Input: part model. Units: mm. Frame: model coordinates. A direction names the side the tool comes from. Give positions to 0.01 mm unless a question says otherwise; leave off trailing zeros. Write each loop counter-clockwise with the first axis right and the second up, starting at its lowest first coordinate (ties: lowest second). Pieces come first, ordered by that corner, then holes. Notation, with made-up numbers: (-33.5, -13.75) - (21.5, -13.75) arc R28 ccw to (21.5, 18.25) - close; hole circle Ø3 at (51.5, 89). An arc over 180 degrees is marked (long way). Answer as CSV lines item,"result". Start each with the question number.
from build123d import *

# Parameters (mm, degrees)
PAD_DEPTH       = 3.95
PAD001_DEPTH    = 8
SKETCH003_W     = 50
SKETCH003_H     = 9.8
PAD002_DEPTH    = 1.5
CHAMFER_SIZE    = 2.5
CHAMFER001_SIZE = 5
FILLET_R        = 2.5
FILLET001_R     = 0.5


with BuildPart() as part:
    # Sketch → Pad (new body)
    with BuildSketch(Plane.XY):
        Polygon((-45, 19.75), (-45, -19.75), (-24.75, -19.75), (-24.75, -45), (-7.25, -45), (-7.25, 19.75), align=None)
    extrude(amount=PAD_DEPTH)

    # Sketch002 → Pad001 (join)
    with BuildSketch(Plane.XY):
        Polygon((-45, 20), (-55, 20), (-55, 0), (-149, 0), (-149, -70), (-7, -70), (-7, -45), (-45, -45), align=None)
    extrude(amount=PAD001_DEPTH)

    # Sketch003 (on Face7 of Pad001) → Pad002 (join)
    with BuildSketch(Plane.XY.offset(8)):
        with Locations((-114, -55)):
            Rectangle(SKETCH003_W, SKETCH003_H)
    extrude(amount=PAD002_DEPTH)

    # Chamfer
    chamfer_edges = [part.edges().sort_by_distance(p)[0] for p in [
        (-7.25, 19.75, 1.975),
    ]]
    chamfer(chamfer_edges, length=CHAMFER_SIZE)

    # Chamfer001
    chamfer001_edges = [part.edges().sort_by_distance(p)[0] for p in [
        (-55, 20, 4),
    ]]
    chamfer(chamfer001_edges, length=CHAMFER001_SIZE)

    # Fillet
    fillet_edges = [part.edges().sort_by_distance(p)[0] for p in [
        (-55, 0, 4),
        (-149, 0, 4),
        (-149, -70, 4),
        (-7, -70, 4),
    ]]
    fillet(fillet_edges, radius=FILLET_R)

    # Fillet001
    fillet001_edges = [part.edges().sort_by_distance(p)[0] for p in [
        (-114, -59.9, 9.5),
        (-89, -55, 9.5),
        (-114, -50.1, 9.5),
        (-139, -55, 9.5),
    ]]
    fillet(fillet001_edges, radius=FILLET001_R)


solid = part.part
1) Reachability of faces 5 (the flat face through (-101, 0, 4)), 6 (the flat face through (-24.75, -32, 2)), 7 (the flat face through (-27, 19.75, 2)), 8 (the flat face through (-45, -20, 5)), 9 (the flat face through (-26, -5, 3.95)) from +Z, -Z, +X, -X, +Y, -Y: full face, straight path, thin tool, end or side. Return the list, or none.
2) Material intervals for line 1 (X direction, y = -26, z = 2.25); line 2 (Y direction, x = -27.5, z = 0.5); line 3 (Y direction, x = -30.5, z = 4.5), sorted ascending. Write a range as from..to.
3) Contact query for flat-ended pins moving along their axis: P1, Ø3, axis at x = -96.5, z = 7, coming from the +Y side; P2, Ø1.2, axis at y = -15.5, z = 3, coming from the +X side; P3, Ø4.5, axis at x = -32.5, z = 2, coming from the +Y side. Output: stop coordinate, or through.
4) Cut plane D-D on x = -135. Output: boundary loops of the cut face in (y, z), and give its area (3 significant figures).
5) Cut plane B-B on y = -26. Output: boundary loops of the cut face in (x, z), and give its area (3 significant figures).
6) Cut plane C-C on z = 1.75. Output: boundary loops of the cut face in (x, y), and give its area (3 significant figures).
7) Cut plane A-A on x = -37.5. Output: boundary loops of the cut face in (y, z), and give its area (3 significant figures).
8) Pull-direction query (Y, two-part tool) for faces 1 (the flat face through (-79, -70, 4)), 2 (the flat face through (-7, -56, 4)), 3 (the flat face through (-53, 17, 4)), 4 (the flat face through (-35, -19.75, 2)); classes: +Y half, -Y half, draft (parallel to the pull), parting line (faces both ways), or undercut.
Numbers:
1,face 5,"+Z, -Z, -X, +Y"
1,face 6,"+Z, -Z"
1,face 7,"+Z, -Z, +X, +Y"
1,face 8,"+Z"
1,face 9,"+Z, +X, +Y"
2,line 1,"x = -149..-45, -24.75..-7.25"
2,line 2,"y = -70..-45, -19.75..19.75"
2,line 3,"y = -70..-45"
3,P1,"stops at y = 0"
3,P2,"stops at x = -7.25"
3,P3,"stops at y = 19.75"
4,outline,"(-70, 0) - (0, 0) - (0, 8) - (-50.1, 8) - (-50.1, 9) arc R0.5 ccw to (-50.6, 9.5) - (-59.4, 9.5) arc R0.5 ccw to (-59.9, 9) - (-59.9, 8) - (-70, 8) - close"
4,area,"575 mm²"
5,outline,"(-149, 0) - (-45, 0) - (-45, 8) - (-149, 8) - close; (-24.75, 0) - (-7.25, 0) - (-7.25, 3.95) - (-24.75, 3.95) - close"
5,area,"901 mm²"
6,outline,"(-149, -67.5) arc R2.5 ccw to (-146.5, -70) - (-9.5, -70) arc R2.5 ccw to (-7, -67.5) - (-7, -45) - (-7.25, -45) - (-7.25, 17.25) - (-9.75, 19.75) - (-45, 19.75) - (-45, 20) - (-50, 20) - (-55, 15) - (-55, 2.5) arc R2.5 cw to (-57.5, 0) - (-146.5, 0) arc R2.5 ccw to (-149, -2.5) - close; hole (-45, -45) - (-24.75, -45) - (-24.75, -19.75) - (-45, -19.75) - close"
6,area,"10,300 mm²"
7,outline,"(-70, 0) - (-45, 0) - (-45, 8) - (-70, 8) - close; (-19.75, 0) - (19.75, 0) - (19.75, 3.95) - (-19.75, 3.95) - close"
7,area,"356 mm²"
8,face 1,"-Y half"
8,face 2,"draft"
8,face 3,"+Y half"
8,face 4,"undercut"
